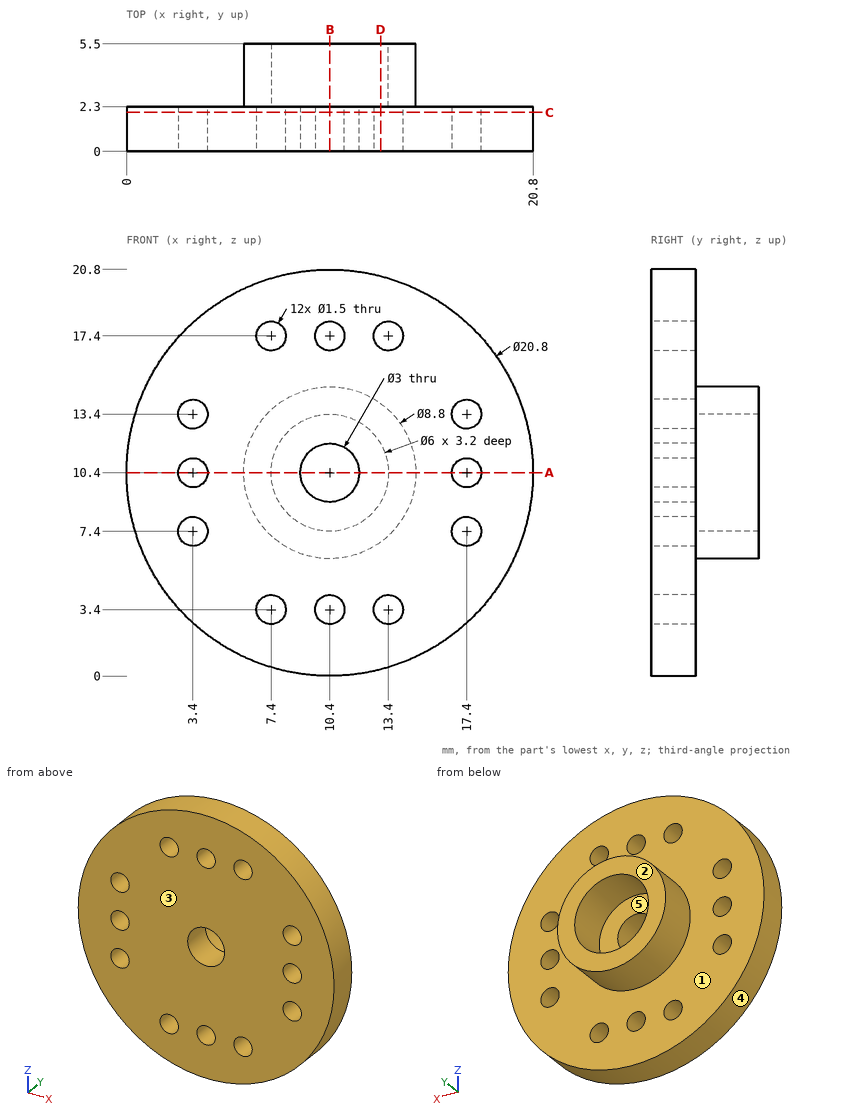
For this review, use the dimensioned drawing (mm, ordinates from the lowest corner) and the shaded views. A direction names the side the tool comes from. Give positions to 0.01 mm unless a question says otherwise; leave off trailing zeros. Order: outer loops, then holes, each group sorted by start corner. A loop starts at its lowest first (then second) coordinate and runs counter-clockwise, first axis right, second up. Notation, with made-up numbers: M 61.25,-21.5 L 87.25,-21.5 A25 ccw 87.25,9.5 Z; hole C 48.5,41 d2. An arc over 180 degrees is marked long. Use one line per item in the form item = value. Start each with the question number.
Item 1: To check wall thickness, follow line 1 along X through (y, z) = (1.45, 7.4); line 2 along X through (y, z) = (1.85, 17.4). State the ranges of each line that lie inside material, in increasing order. Write a range as from..to.
Item 2: The part is to be moulded in two halves that separate along Z. For the marked faces 3, 4 and 5, say which applies: pulls with the +Z half, pulls with the -Z half, needs draft (parallel to the pull), parting line crosses it, or undercut.
Item 3: For the marked faces 1 and 2, list the 3-axis set-ups (+Z, -Z, +X, -X, +Y, -Y) from which the entire face can be reached by the end or side of a thin tool; tool diameter is ignored.
Item 4: We need section B-B on x = 10.4. Give the boundary of the cut face in (y, z).
Item 5: Insertion check: pin 1 Ø1.4 at (x, z) = (10.4, 3.4) entering from -Y; pin 2 Ø2.5 at (x, z) = (13.4, 3.4) entering from +Y; pin 3 Ø2 at (x, y) = (9, 4.5) entering from -Z; pin 4 Ø1 at (x, y) = (13.5, 3.5) entering from -Z. Each pin has a flat end and moves straight along its axis. Give the tip position at first contact, or say it passes through.
Item 6: We need section D-D on x = 13. Give the boundary of the cut face in (y, z).
Item 7: We need section A-A on z = 10.4. Give the boundary of the cut face in (x, y), plus the area to 3 significant figures.
Item 8: We need section C-C on y = 2. Give the number of separate pieces and of enclosed holes in the cut face, plus the area to 3 significant figures.
Completed:
q1.line_1 = 0.44..2.65, 4.15..16.65, 18.15..20.36
q1.line_2 = 2.71..6.65, 8.15..9.65, 11.15..12.65, 14.15..18.09
q2.face_3 = needs draft
q2.face_4 = parting line crosses it
q2.face_5 = undercut
q3.face_1 = +Y
q3.face_2 = +Z, -Z, +X, -X, +Y
q4.outline = M 0,0 L 2.3,0 L 2.3,2.65 L 0,2.65 Z; M 0,4.15 L 2.3,4.15 L 2.3,6 L 5.5,6 L 5.5,7.4 L 2.3,7.4 L 2.3,8.9 L 0,8.9 Z; M 0,11.9 L 2.3,11.9 L 2.3,13.4 L 5.5,13.4 L 5.5,14.8 L 2.3,14.8 L 2.3,16.65 L 0,16.65 Z; M 0,18.15 L 2.3,18.15 L 2.3,20.8 L 0,20.8 Z
q5.pin_1 = through
q5.pin_2 = 2.3
q5.pin_3 = 6.02
q5.pin_4 = 6.85
q6.outline = M 0,0.33 L 2.3,0.33 L 2.3,2.77 L 0,2.77 Z; M 0,4.03 L 2.3,4.03 L 2.3,6.85 L 5.5,6.85 L 5.5,8.9 L 2.3,8.9 L 2.3,11.9 L 5.5,11.9 L 5.5,13.95 L 2.3,13.95 L 2.3,16.77 L 0,16.77 Z; M 0,18.03 L 2.3,18.03 L 2.3,20.47 L 0,20.47 Z
q7.outline = M 0,0 L 2.65,0 L 2.65,2.3 L 0,2.3 Z; M 4.15,0 L 8.9,0 L 8.9,2.3 L 7.4,2.3 L 7.4,5.5 L 6,5.5 L 6,2.3 L 4.15,2.3 Z; M 11.9,0 L 16.65,0 L 16.65,2.3 L 14.8,2.3 L 14.8,5.5 L 13.4,5.5 L 13.4,2.3 L 11.9,2.3 Z; M 18.15,0 L 20.8,0 L 20.8,2.3 L 18.15,2.3 Z
q7.area = 43.0 mm²
q8.separate_pieces = 1
q8.enclosed_holes = 13
q8.area = 312 mm²
